Geometry check sheet. Reference: the model listing, model coordinates, mm. A direction names the side the tool comes from. Round coordinates to 2 decimals unless told otherwise and drop trailing zeros. Order: outer loops, then holes, each group sorted by start corner. A loop starts at its lowest first (then second) coordinate and runs counter-clockwise, first axis right, second up. Notation, with made-up numbers: M 47.25,52.25 L 77.25,52.25 A26 cw 77.25,79.25 Z; hole C 1.5,-20.75 d10. An arc over 180 degrees is marked long. Return JSON: item names as keys, results as strings. Group by question number.
```python
from build123d import *

# Parameters (mm, degrees)
SKETCH1_R               = 12.065
BOSS_EXTRUDE1_DEPTH     = 10.795
SKETCH5_W               = 38.1
SKETCH5_H               = 21.59
BOSS_EXTRUDE2_DEPTH     = 101.6
CUT_EXTRUDE1_REACH      = 261.255
SKETCH6_R               = 3.175
SKETCH4_W               = 12.7
SKETCH4_H               = 21.59
BOSS_EXTRUDE3_DEPTH     = 50.8
CUT_EXTRUDE2_DEPTH      = 210.73176208
CUT_EXTRUDE2_DEPTH_BACK = 210.73176208
SKETCH6_2_R             = 3.175
CUT_EXTRUDE3_DEPTH      = 214.164307578
CUT_EXTRUDE3_DEPTH_BACK = 214.164307578
CUT_EXTRUDE4_DEPTH      = 200.616791257
CUT_EXTRUDE4_DEPTH_BACK = 200.616791257


with BuildPart() as part:
    # Sketch1 → Boss-Extrude1 (new, symmetric)
    with BuildSketch(Plane(origin=(0, 0, 0), x_dir=(1, 0, 0), z_dir=(0, 1, 0))):
        with BuildLine():
            Line((-31.75, 152.4), (31.75, 152.4))
            ThreePointArc((31.75, 152.4), (21.755106695, 76.491146914), (18.415, 0))
            ThreePointArc((18.415, 0), (0, -18.415), (-18.415, 0))
            ThreePointArc((-18.415, 0), (-21.755106695, 76.491146914), (-31.75, 152.4))
        make_face()
        with Locations(Location((0, 0, 0), (0, 0, 270))):
            Circle(SKETCH1_R, mode=Mode.SUBTRACT)
    extrude(amount=BOSS_EXTRUDE1_DEPTH, both=True)

    # Sketch5 → Boss-Extrude2 (add)
    with BuildSketch(Plane(origin=(0, 0, -152.4), x_dir=(-1, 0, 0), z_dir=(0, 0, -1))):
        Rectangle(SKETCH5_W, SKETCH5_H)
    extrude(amount=BOSS_EXTRUDE2_DEPTH)

    # Sketch6 → Cut-Extrude1 (cut, up to next)
    with BuildSketch(Plane(origin=(19.05, 0, 0), x_dir=(0, 0, -1), z_dir=(1, 0, 0)), mode=Mode.PRIVATE) as cut_extrude1_sk1:
        Polygon((152.4, -10.795), (154.288880246, 10.795), (254, 10.795), (254, -10.795), align=None)
        with Locations((185.094440123, 0)):
            Circle(SKETCH6_R, mode=Mode.SUBTRACT)
    cut_extrude1_tool1 = extrude(cut_extrude1_sk1.sketch, amount=-CUT_EXTRUDE1_REACH, mode=Mode.PRIVATE) & part.part
    add(cut_extrude1_tool1.solids().sort_by_distance((19.05, -0.034262, -203.945458))[0], mode=Mode.SUBTRACT)


with BuildPart() as cut_extrude1_piece_1:
    # of the separate pieces the step leaves, piece 1, a body of its own (cut_extrude1_pieces)
    add(part.part.solids().sort_by_distance((-31.75, -10.795, -152.4))[0])

    # Sketch4 → Boss-Extrude3 (add)
    with BuildSketch(Plane(origin=(0, 0, -152.4), x_dir=(-1, 0, 0), z_dir=(0, 0, -1))):
        with Locations((25.4, 0)):
            Rectangle(SKETCH4_W, SKETCH4_H)
        with Locations((-25.4, 0)):
            Rectangle(SKETCH4_W, SKETCH4_H)
    extrude(amount=BOSS_EXTRUDE3_DEPTH)


with BuildPart() as cut_extrude1_piece_2:
    # of the separate pieces the step leaves, piece 2, a body of its own (cut_extrude1_pieces)
    add(part.part.solids().sort_by_distance((-19.05, 0, -188.269440123))[0])


with BuildPart() as cut_extrude2_tool:
    # Sketch6_2 → Cut-Extrude2 (new, two sides: drawn at the far end of the back side and taken through both)
    with BuildSketch(Plane(origin=(19.05, 0, 0), x_dir=(0, 0, -1), z_dir=(1, 0, 0)).offset(-CUT_EXTRUDE2_DEPTH_BACK)):
        with Locations((185.094440123, 0)):
            Circle(SKETCH6_2_R)
    extrude(amount=CUT_EXTRUDE2_DEPTH + CUT_EXTRUDE2_DEPTH_BACK)


with BuildPart() as cut_extrude1_piece_1_1:
    add(cut_extrude1_piece_1.part)

    # Cut-Extrude2: cut by cut_extrude2_tool
    add(cut_extrude2_tool.part, mode=Mode.SUBTRACT)

    # Sketch7 → Cut-Extrude3 (cut, two sides: drawn at the far end of the back side and taken through both)
    with BuildSketch(Plane(origin=(31.75, 0, 0), x_dir=(0, 0, -1), z_dir=(1, 0, 0)).offset(-CUT_EXTRUDE3_DEPTH_BACK)):
        with BuildLine():
            Line((203.2, 10.795), (185.094440123, 10.795))
            ThreePointArc((185.094440123, 10.795), (192.727657826, 7.633217703), (195.889440123, 0))
            ThreePointArc((195.889440123, 0), (192.727657826, -7.633217703), (185.094440123, -10.795))
            Line((185.094440123, -10.795), (203.2, -10.795))
            Line((203.2, -10.795), (203.2, 10.795))
        make_face()
    extrude(amount=CUT_EXTRUDE3_DEPTH + CUT_EXTRUDE3_DEPTH_BACK, mode=Mode.SUBTRACT)

    # Sketch8 → Cut-Extrude4 (cut, two sides: drawn at the far end of the back side and taken through both)
    with BuildSketch(Plane.XZ.offset(10.795).offset(-CUT_EXTRUDE4_DEPTH_BACK)):
        with BuildLine():
            ThreePointArc((-10.919216068, -14.828450541), (-14.419629325, -80.021900258), (-22.715851164, -144.78))
            Line((-22.715851164, -144.78), (22.715851164, -144.78))
            ThreePointArc((22.715851164, -144.78), (14.419629325, -80.021900258), (10.919216068, -14.828450541))
            ThreePointArc((10.919216068, -14.828450541), (0, -18.415), (-10.919216068, -14.828450541))
        make_face()
    extrude(amount=CUT_EXTRUDE4_DEPTH + CUT_EXTRUDE4_DEPTH_BACK, mode=Mode.SUBTRACT)


with BuildPart() as cut_extrude1_piece_2_1:
    add(cut_extrude1_piece_2.part)

    # Cut-Extrude2: cut by cut_extrude2_tool
    add(cut_extrude2_tool.part, mode=Mode.SUBTRACT)


solid = cut_extrude1_piece_1_1.part
```
Q1. Section check C-C on y = -8.25. Record the cut outline in (x, z) (3 decimals), plus the area to 3 significant figures.
Q2. Material ranges on line 1 along X through (y, z) = (-4, -160.5); line 2 along Z through (x, y) = (-7, 2); line 3 along Z through (x, y) = (-9, 7), recorded low to high.
Q3. Section check B-B on x = 0. Record the cut outline in (y, z) (3 decimals), plus the area to 3 significant figures.
Q4. Section check A-A on z = -168. Record the cut outline in (x, y) (3 decimals).
Q5. Set-up check for faces 1 (the face through (-21, 10.795, -105)), 2 (the face through (-14.337, 0.151, -79.111)), 3 (the face through (0.27, -0.15, -153.33)): record each of +Z, -Z, +X, -X, +Y, -Y from which the full face is reachable in a straight line by a thin tool's end or side.
Q6. Release check for a two-part mould opening along Z. For faces 4 (the face through (-31.75, 0, -174)), 5 (the face through (21.85, 0.15, -77.56)), 6 (the face through (0.164, 0.151, -18.414)) record: +Z half, -Z half, draft (parallel to the pull), parting line (faces both ways), or undercut.
Q7. Depth check by flat-ended pin: pin 1 Ø8 at (x, y) = (4, 4) entering from +Z (3 decimals); pin 2 Ø5 at (y, z) = (0, -185.09) entering from -X; pin 3 Ø10 at (y, z) = (3, -5) entering from -X; pin 4 Ø3 at (x, y) = (2, 7.5) entering from -Z. Enter the tip coordinate at first touch or a pass-through.
Geometry check:
{
 "1": {"outline": "M -31.75,-192.056 L -19.05,-192.056 L -19.05,-152.623 L 19.05,-152.623 L 19.05,-192.056 L 31.75,-192.056 L 31.75,-152.4 A877.525 cw 18.415,0 A18.415 ccw -18.415,0 A877.525 cw -31.75,-152.4 Z; hole M -22.716,-144.78 L 22.716,-144.78 A885.145 cw 10.919,-14.828 A18.415 cw -10.919,-14.828 A885.145 cw Z; hole C 0,0 d24.13", "area": "4,160 mm^2"},
 "2": {"line 1": "x = -31.75 to -19.05, 19.05 to 31.75", "line 2": "z = -153.52 to -144.78, -17.03 to -9.83, 9.83 to 17.03", "line 3": "z = -153.96 to -144.78, -16.07 to -8.04, 8.04 to 16.07"},
 "3": {"outline": "M -10.795,-152.4 L 10.795,-154.289 L 10.795,-144.78 L -10.795,-144.78 Z; M -10.795,-18.415 L 10.795,-18.415 L 10.795,-12.065 L -10.795,-12.065 Z; M -10.795,12.065 L 10.795,12.065 L 10.795,18.415 L -10.795,18.415 Z", "area": "459 mm^2"},
 "4": {"outline": "M -31.75,-10.795 L -19.05,-10.795 L -19.05,10.795 L -31.75,10.795 Z; M 19.05,-10.795 L 31.75,-10.795 L 31.75,10.795 L 19.05,10.795 Z"},
 "5": {"face 1": "+Z, -Z, +X, -X, +Y", "face 2": "+Y, -Y", "face 3": "-Z, -Y"},
 "6": {"face 4": "draft", "face 5": "+Z half", "face 6": "undercut"},
 "7": {"pin 1": "stops at z = 18.415", "pin 2": "passes through", "pin 3": "stops at x = -18.47", "pin 4": "stops at z = -154.13"}
}
